from build123d import *

# Parameters (mm, degrees)
SKETCH1_R          = 19.05
BASE_EXTRUDE_DEPTH = 3.175


with BuildPart() as part:
    # Sketch1 → Base-Extrude (new body)
    with BuildSketch(Plane.XY):
        with BuildLine():
            Line((-752.475, -95.262203185), (-684.4284, -359.69737999))
            ThreePointArc((-684.4284, -359.69737999), (0.19670941, -273.050007044), (684.8094, -359.795448169))
            Line((684.8094, -359.795448169), (752.475, -95.262203185))
            ThreePointArc((752.475, -95.262203185), (0, 0), (-752.475, -95.262203185))
        make_face()
        with Locations((-444.0174, -113.4618)):
            Circle(SKETCH1_R, mode=Mode.SUBTRACT)
        with BuildLine():
            Line((-535.614695533, -127.743373783), (-532.38464705, -199.45456113))
            add(Edge.make_bspline(
                [(-532.38464705, -199.45456113), (-528.480595277, -286.129479355), (-464.930974485, -261.798673459), (-401.381353693, -237.467867563), (-456.359855014, -170.347472288)],
                knots=[4.298855998, 4.298855998, 4.298855998, 6.283185307, 6.283185307, 8.267514616, 8.267514616, 8.267514616], degree=2, weights=[1, 0.546878869, 1, 0.546878869, 1]))
            Line((-456.359855014, -170.347472288), (-501.846758135, -114.814876019))
            ThreePointArc((-501.846758135, -114.814876019), (-523.395377478, -109.095526016), (-535.614695533, -127.743373783))
        make_face(mode=Mode.SUBTRACT)
    extrude(amount=-BASE_EXTRUDE_DEPTH)


solid = part.part
Geometry check sheet. Reference: the model listing, model coordinates, mm. Round coordinates to 2 decimals unless told otherwise and drop trailing zeros. Loops run counter-clockwise (first coordinate to the right, second up) from the corner with the lowest first, then second, coordinate; pieces in that order, holes last. Notation, with made-up numbers: (23, 32.5) -> (55, 32.5) arc R27 ccw to (55, 68.5) -> close; hole circle Ø5 at (-17, -9.75). An arc over 180 degrees is marked (long way). Answer as a JSON object with one key per item and string values. Group by question number.
Item 1: Depth check by flat-ended pin: pin 1 Ø1.5 at (y, z) = (-101.5, -2.5) entering from -X. Enter the tip coordinate at first touch or a pass-through.
Item 2: Thickness scan on line 1 along X through (y, z) = (-245.5, -1.05); line 2 along X through (y, z) = (-219.5, -2.25); line 3 along X through (y, z) = (-131, -2.25). Record the ranges inside material, lowest first.
Item 3: Cross-section at A-A, the plane y = -327. Record the cut outline in (x, z) (3 decimals), plus the area to 3 significant figures.
Item 4: Release check for a two-part mould opening along Y. For faces 1 (the face through (-459.1, -125.1, -1.6)), 2 (the face through (-478.785, -142.97, -1.565)), 3 (the face through (-11, -177, 0)), 4 (the face through (-718.928, -225.629, -1.565)) record: pulls with the +Y half, pulls with the -Y half, needs draft (parallel to the pull), parting line crosses it, or undercut.
Item 5: Cross-section at B-B, the plane x = -179.5. Record the cut outline in (y, z) (3 decimals).
Item 6: Cross-section at D-D, the plane z = -2.2. Count the separate pieces of the cut face and the enclosed holes in it, plus the area to 3 significant figures.
Determined:
{
 "1": {"pin 1": "stops at x = -751.06"},
 "2": {"line 1": "x = -713.81 to -513.84, -446.39 to 714.05", "line 2": "x = -720.51 to -528.64, -439.44 to 720.7", "line 3": "x = -743.28 to -535.47, -488.59 to -451.45, -436.58 to 743.33"},
 "3": {"outline": "(-692.842, -3.175) -> (-541.696, -3.175) -> (-541.696, 0) -> (-692.842, 0) -> close; (541.696, -3.175) -> (693.198, -3.175) -> (693.198, 0) -> (541.696, 0) -> close", "area": "961 mm²"},
 "4": {"face 1": "undercut", "face 2": "undercut", "face 3": "needs draft", "face 4": "pulls with the -Y half"},
 "5": {"outline": "(-278.922, -3.175) -> (-5.34, -3.175) -> (-5.34, 0) -> (-278.922, 0) -> close"},
 "6": {"separate pieces": "1", "enclosed holes": "2", "area": "385,000 mm²"}
}
